```python
from build123d import *

# Parameters (mm, degrees)
SKETCH1_W           = 84.61
SKETCH1_H           = 24
BOSS_EXTRUDE1_DEPTH = 3.18
SKETCH10_W          = 24
SKETCH10_H          = 3.18
BOSS_EXTRUDE2_DEPTH = 2
SKETCH9_W           = 3.28
SKETCH9_H           = 12.15
CUT_EXTRUDE1_DEPTH  = 61.496753834


with BuildPart() as part:
    # Sketch1 → Boss-Extrude1 (new body)
    with BuildSketch(Plane(origin=(0, 0, 0), x_dir=(1, 0, 0), z_dir=(0, 1, 0))):
        with Locations((-13.483376754, -5.613867735)):
            Rectangle(SKETCH1_W, SKETCH1_H)
    extrude(amount=BOSS_EXTRUDE1_DEPTH)

    # Sketch10 → Boss-Extrude2 (add)
    with BuildSketch(Plane.ZY.offset(55.788376754)):
        with Locations((5.613867735, 1.59)):
            Rectangle(SKETCH10_W, SKETCH10_H)
    boss_extrude2 = extrude(amount=BOSS_EXTRUDE2_DEPTH)

    # Sketch9 → Cut-Extrude1 (cut, through all)
    with BuildSketch(Plane(origin=(0, 3.18, 0), x_dir=(1, 0, 0), z_dir=(0, 1, 0))):
        with Locations((-54.148376754, -5.613867735)):
            Rectangle(SKETCH9_W, SKETCH9_H)
    cut_extrude1 = extrude(amount=-CUT_EXTRUDE1_DEPTH, mode=Mode.SUBTRACT)

    # Mirror1: Boss-Extrude2, Cut-Extrude1 across plane
    add(boss_extrude2.mirror(Plane.ZY.offset(13.483376754)))
    add(cut_extrude1.mirror(Plane.ZY.offset(13.483376754)), mode=Mode.SUBTRACT)


solid = part.part
```
Could you check a few things on this model? Use its own coordinates, in mm. A direction names the side the tool comes from. Coordinates: 2 decimals unless noted, no trailing zeros. Write each loop counter-clockwise with the first axis right and the second up, starting at its lowest first coordinate (ties: lowest second). Pieces come first, ordered by that corner, then holes. Notation, with made-up numbers: (74.25, 49) -> (84.25, 49) arc R4 ccw to (84.25, 56) -> close; hole circle Ø6 at (87.5, 41.5). An arc over 180 degrees is marked (long way). One line per question, with ' | ' between items. Start each with the question number.
1. If we section it at A-A (z = 4): Please give me the cut outline in (x, y).
2. For faces 1 (the face through (-55.788, 2, 6)), 2 (the face through (-14, 0, 5)), which set-ups out of +Z, -Z, +X, -X, +Y, -Y let a thin tool reach every point of the face, with its end or its side?
3. Will this pin go through, and if not, where does the flat tip stop? P1, Ø12, axis at x = -36, z = -2, coming from the -Y side.
4. Please list where this line runs through material, in increasing order: line 1 along X through (y, z) = (0.25, 4.75).
5. If we section it at B-B (y = 0.9): Please give me the cut outline in (x, z).
6. Thinking about a two-plate mould opening in Z: for faces 3 (the face through (30.822, 2, 5)), 4 (the face through (-14, 2, 17.614)), 5 (the face through (-54, 2, 11.689)), which applies, pulls with the +Z half, pulls with the -Z half, needs draft (parallel to the pull), parting line crosses it, or undercut?
Return value:
1) outline: (-57.79, 0) -> (-55.79, 0) -> (-55.79, 3.18) -> (-57.79, 3.18) -> close; (-52.51, 0) -> (25.54, 0) -> (25.54, 3.18) -> (-52.51, 3.18) -> close; (28.82, 0) -> (30.82, 0) -> (30.82, 3.18) -> (28.82, 3.18) -> close
2) face 1: +Y, -Y | face 2: +Z, -Z, +X, -X, -Y
3) P1: stops at y = 0
4) line 1: x = -57.79 to -55.79, -52.51 to 25.54, 28.82 to 30.82
5) outline: (-57.79, -6.39) -> (30.82, -6.39) -> (30.82, 17.61) -> (-57.79, 17.61) -> close; hole (-55.79, -0.46) -> (-52.51, -0.46) -> (-52.51, 11.69) -> (-55.79, 11.69) -> close; hole (25.54, -0.46) -> (28.82, -0.46) -> (28.82, 11.69) -> (25.54, 11.69) -> close
6) face 3: needs draft | face 4: pulls with the +Z half | face 5: undercut
